The listing builds one solid part. Answer for the finished solid, in the listing's coordinates (mm). A direction names the side the tool comes from. Coordinates: 2 decimals unless noted, no trailing zeros. Order: outer loops, then holes, each group sorted by start corner. A loop starts at its lowest first (then second) coordinate and runs counter-clockwise, first axis right, second up. Notation, with made-up numbers: (4.25, 19) - (42.25, 19) arc R21 ccw to (42.25, 34) - close; hole circle Ø2 at (44, 45.25). An arc over 180 degrees is marked (long way). Use one line per item in the form item = value. Start each with the question number.
Item 1: A tool of negligible diameter and unlimited length cuts with its end or side. For faces 1 (the cylindrical face through (-13.69, 119.48, 8.41)), 2 (the cylindrical face through (-0.9, 119.14, 5.36)), 3 (the flat face through (-70, 20, 4)), from which of +Z, -Z, +X, -X, +Y, -Y can it reach the whole face along a straight path? Write none if from no direction.
Item 2: Each of these flat-tipped pins is pushed along its axis until it touches: pin 1 Ø1.7 at (y, z) = (65, 3.5) entering from -X; pin 2 Ø5 at (x, z) = (-70, 8) entering from +Y; pin 3 Ø0.7 at (x, z) = (-79, 9) entering from +Y. Where does it stop, or does it pass through?
Item 3: Section A-A, the plane x = -39 is taken. Write down the section's boundary in (y, z).
Item 4: Section B-B, the plane y = 107 is taken. Write down the section's boundary in (x, z).
Item 5: Consider line 1 along Y through (x, z) = (-15, 6.25); line 2 along X through (y, z) = (15, 5.75); line 3 along Y through (x, z) = (-26.5, 5.25). Determine where each line is inside the solid, lowest interval first. Write a range as [from, to].
from build123d import *

# Parameters (mm, degrees)
F1_DEPTH = 8
F3_DEPTH = 1.4
F4_R     = 3
F5_DEPTH = 9.401
F6_R     = 5
F7_R     = 3
F8_SIZE  = 1.2
F9_SIZE  = 1.2


with BuildPart() as f1:
    # F0 (on Top) → F1 (new body)
    with BuildSketch(Plane.XY):
        Polygon((0, 0), (0, 120), (-20, 120), (-20, 20), (-120, 20), (-120, 0), align=None)
    extrude(amount=F1_DEPTH)

    # F2 (on face) → F3 (join)
    with BuildSketch(Plane.XY.offset(8)):
        Polygon((-120, 0), (0, 0), (0, 120), (-15, 120), (-15, 15), (-120, 15), align=None)
    extrude(amount=F3_DEPTH)

    # F4 (on face) → F5 (cut, through all)
    with BuildSketch(Plane.XY.offset(9.4)):
        with Locations((-15, 15)):
            Circle(F4_R)
    extrude(amount=-F5_DEPTH, mode=Mode.SUBTRACT)

    # F6
    f6_edges = [f1.edges().sort_by_distance(p)[0] for p in [
        (-20, 20, 4),
    ]]
    fillet(f6_edges, radius=F6_R)

    # F7
    f7_edges = [f1.edges().sort_by_distance(p)[0] for p in [
        (0, 0, 4.7),
        (0, 120, 4.7),
        (-20, 120, 4),
        (-120, 20, 4),
        (-120, 0, 4.7),
        (-120, 15, 8.7),
        (-15, 18, 8.7),
        (-18, 15, 8.7),
        (-15, 120, 8.7),
    ]]
    fillet(f7_edges, radius=F7_R)

    # F8
    f8_edges = [f1.edges().sort_by_distance(p)[0] for p in [
        (-20, 71, 8),
    ]]
    chamfer(f8_edges, length=F8_SIZE)

    # F9
    f9_edges = [f1.edges().sort_by_distance(p)[0] for p in [
        (-60, 0, 0),
        (-18, 15, 0),
    ]]
    chamfer(f9_edges, length=F9_SIZE)


solid = f1.part
Response:
q1.face_1 = +Z, -X, +Y
q1.face_2 = +Z, -Z, +X, +Y
q1.face_3 = +Z, -Z, -X, +Y
q2.pin_1 = -20
q2.pin_2 = 20
q2.pin_3 = 15
q3.outline = (0, 1.2) - (1.2, 0) - (18.8, 0) - (20, 1.2) - (20, 6.8) - (18.8, 8) - (15, 8) - (15, 9.4) - (0, 9.4) - close
q4.outline = (-20, 1.2) - (-18.8, 0) - (-1.2, 0) - (0, 1.2) - (0, 9.4) - (-15, 9.4) - (-15, 8) - (-18.8, 8) - (-20, 6.8) - close
q5.line_1 = [0, 12], [18, 120]
q5.line_2 = [-120, -18], [-12, 0]
q5.line_3 = [0, 20]
